Autodesk Inventor part; units mm, degrees
ref_plane "YZ Plane" through (0, 0, 0) normal (1, 0, 0) x (0, 1, 0)
ref_plane "XZ Plane" through (0, 0, 0) normal (0, 1, 0) x (-1, 0, 0)
ref_plane "XY Plane" through (0, 0, 0) normal (0, 0, 1) x (1, 0, 0)
sketch "Boceto1" plane through (0, 0, 0) normal (0, 0, 1) x (1, 0, 0)
  line L0 (0, 0) -> (127.5, 0)
  line L1 (127.5, 0) -> (127.5, 177)
  line L2 (127.5, 177) -> (0, 177)
  line L3 (0, 177) -> (0, 0)
  dimension "d32" = 127.5
  dimension "d33" = 177
extrude "Extrusión1" add sketch "Boceto1" along normal blind 6
ref_plane "Plano de trabajo6" through (0, 88.5, 0) normal (0, -1, 0) x (1, 0, 0)
ref_plane "Plano de trabajo7" through (63.75, 0, 0) normal (-1, 0, 0) x (0, 0, 1)
sketch "Boceto17" plane through (0, 0, 6) normal (0, 0, 1) x (1, 0, 0)
  line L0 (127.5, 0) -> (116, 0)
  line L1 (116, 0) -> (116, 11.5)
  line L2 (116, 11.5) -> (127.5, 11.5)
  line L3 (127.5, 11.5) -> (127.5, 0)
  line L4 (0, 0) -> (11.5, 0)
  line L5 (11.5, 0) -> (11.5, 11.5)
  line L6 (11.5, 11.5) -> (0, 11.5)
  line L7 (0, 11.5) -> (0, 0)
  line L8 (127.5, 177) -> (116, 177)
  line L9 (116, 177) -> (116, 165.5)
  line L10 (116, 165.5) -> (127.5, 165.5)
  line L11 (127.5, 165.5) -> (127.5, 177)
  line L12 (0, 177) -> (11.5, 177)
  line L13 (11.5, 177) -> (11.5, 165.5)
  line L14 (11.5, 165.5) -> (0, 165.5)
  line L15 (0, 165.5) -> (0, 177)
  dimension "d124" = 11.5
  dimension "d125" = 11.5
  dimension "d129" = 11.5
  dimension "d130" = 11.5
  dimension "d131" = 11.5
  dimension "d132" = 11.5
  dimension "d133" = 11.5
  dimension "d134" = 11.5
extrude "Extrusión12" cut sketch "Boceto17" against normal blind 4
sketch "Boceto18" plane through (0, 0, 2) normal (0, 0, 1) x (1, 0, 0)
  line L0 (0, 0) -> (11.5, 0)
  line L1 (11.5, 0) -> (11.5, 11.5)
  line L2 (11.5, 11.5) -> (0, 11.5)
  line L3 (0, 11.5) -> (0, 0)
  line L4 (127.5, 0) -> (116, 0)
  line L5 (116, 0) -> (116, 11.5)
  line L6 (116, 11.5) -> (127.5, 11.5)
  line L7 (127.5, 11.5) -> (127.5, 0)
  line L8 (127.5, 177) -> (116, 177)
  line L9 (116, 177) -> (116, 165.5)
  line L10 (116, 165.5) -> (127.5, 165.5)
  line L11 (127.5, 165.5) -> (127.5, 177)
  line L12 (0, 177) -> (11.5, 177)
  line L13 (11.5, 177) -> (11.5, 165.5)
  line L14 (11.5, 165.5) -> (0, 165.5)
  line L15 (0, 165.5) -> (0, 177)
  line L16 (116, 11.5) -> (127.5, 0)
  line L17 (127.5, 11.5) -> (116, 0)
  circle A0 centre (121.75, 5.75) radius 2
  dimension "d137" = 4
extrude "Extrusión13" cut sketch "Boceto18" against normal blind 3.2 contours A0 L17 L16 | L16 L17 A0 | A0 L16 L17 | L17 L16 A0
mirror "Simetría7" about plane through (63.75, 0, 0) normal (-1, 0, 0) of "Extrusión13"
mirror "Simetría8" about plane through (0, 88.5, 0) normal (0, -1, 0) of "Extrusión13", "Simetría7"
sketch "Boceto19" plane through (0, 0, 6) normal (0, 0, 1) x (1, 0, 0)
  line L0 (0, 0) -> (127.5, 0)
  line L1 (127.5, 0) -> (127.5, 85.5)
  line L2 (127.5, 85.5) -> (0, 85.5)
  line L3 (0, 85.5) -> (0, 0)
  line L4 (127.5, 0) -> (127.5, 177)
  line L5 (0, 85.5) -> (127.5, 85.5)
  line L6 (127.5, 85.5) -> (127.5, 91.5)
  line L7 (127.5, 91.5) -> (0, 91.5)
  line L8 (0, 91.5) -> (0, 85.5)
  line L9 (0, 91.5) -> (127.5, 91.5)
  line L10 (127.5, 91.5) -> (127.5, 177)
  line L11 (127.5, 177) -> (0, 177)
  line L12 (0, 177) -> (0, 91.5)
  dimension "d140" = 127.5
  dimension "d141" = 85.5
  dimension "d142" = 6
extrude "Extrusión14" cut sketch "Boceto19" against normal blind 4.2 contours L8 L7 L4 L2
properties part number "transillum_diffusor_partC_v1"
The listing builds one solid part. Answer for the finished solid, in the listing's coordinates (mm). A direction names the side the tool comes from. Give positions to 0.01 mm unless a question says otherwise; leave off trailing zeros. Write each loop counter-clockwise with the first axis right and the second up, starting at its lowest first coordinate (ties: lowest second). Pieces come first, ordered by that corner, then holes. Notation, with made-up numbers: (-21.75, -28) -> (3.25, -28) arc R17 ccw to (3.25, -22) -> close; hole circle Ø10 at (14.25, 0). An arc over 180 degrees is marked (long way). Use one line per item in the form item = value.
1) Section A-A on z = 4.8 is taken. Write down the section's boundary in (x, y), plus the area to 3 significant figures.
Result:
outline = (0, 11.5) -> (11.5, 11.5) -> (11.5, 0) -> (116, 0) -> (116, 11.5) -> (127.5, 11.5) -> (127.5, 85.5) -> (0, 85.5) -> close; (0, 91.5) -> (127.5, 91.5) -> (127.5, 165.5) -> (116, 165.5) -> (116, 177) -> (11.5, 177) -> (11.5, 165.5) -> (0, 165.5) -> close
area = 21,300 mm²
2) Each of these flat-tipped pins is pushed along its axis until it touches: P1, Ø2.5, axis at x = 121.75, y = 5.75, coming from the -Z side; P2, Ø2, axis at y = 172, z = 5, coming from the +X side; P3, Ø3, axis at x = 65, y = 111.5, coming from the -Z side; P4, Ø3.5, axis at x = 124, y = 8, coming from the +Z side. Where does it stop, or does it pass through?
Result:
P1 = through
P2 = 116
P3 = 0
P4 = 2
3) For a pull along Y with two mould halves and no side action, classify faces 1 (the flat face through (122, 165.5, 4)), 2 (the flat face through (119, 171, 2)), 3 (the flat face through (63, 89, 1.8)), 4 (the cylindrical face through (119.752, 5.838, 1.014)) as +Y half, -Y half, draft (parallel to the pull), parting line (faces both ways), or undercut.
Result:
face_1 = +Y half
face_2 = draft
face_3 = undercut
face_4 = undercut
4) Section C-C on x = 121.75 is taken. Write down the section's boundary in (y, z), plus the area to 3 significant figures.
Result:
outline = (0, 0) -> (3.75, 0) -> (3.75, 2) -> (0, 2) -> close; (7.75, 0) -> (169.25, 0) -> (169.25, 2) -> (165.5, 2) -> (165.5, 6) -> (91.5, 6) -> (91.5, 1.8) -> (85.5, 1.8) -> (85.5, 6) -> (11.5, 6) -> (11.5, 2) -> (7.75, 2) -> close; (173.25, 0) -> (177, 0) -> (177, 2) -> (173.25, 2) -> close
area = 929 mm²
5) Section B-B on y = 5.75 is taken. Write down the section's boundary in (x, z).
Result:
outline = (0, 0) -> (3.75, 0) -> (3.75, 2) -> (0, 2) -> close; (7.75, 0) -> (119.75, 0) -> (119.75, 2) -> (116, 2) -> (116, 6) -> (11.5, 6) -> (11.5, 2) -> (7.75, 2) -> close; (123.75, 0) -> (127.5, 0) -> (127.5, 2) -> (123.75, 2) -> close
6) A tool of negligible diameter and unlimited length cuts with its end or side. For faces 5 (the flat face through (6, 11.5, 4)), 6 (the flat face through (6, 165.5, 4)), 7 (the flat face through (122, 11.5, 4)), 8 (the flat face through (65, 85.5, 4)), from which of +Z, -Z, +X, -X, +Y, -Y can it reach the whole face along a straight path? Write none if from no direction.
Result:
face_5 = +Z, -X, -Y
face_6 = +Z, -X, +Y
face_7 = +Z, +X, -Y
face_8 = +Z, +X, -X
7) Straight lines are drawn through the part: probe 1 along X at (y, z) = (171.25, 0.95); probe 2 along Y at (x, z) = (121.75, 0.7); probe 3 along Y at (x, z) = (39.5, 2.95). For each, find the intervals that lie inside material, in ascending order.
Result:
probe_1 = 0 to 3.75, 7.75 to 119.75, 123.75 to 127.5
probe_2 = 0 to 3.75, 7.75 to 169.25, 173.25 to 177
probe_3 = 0 to 85.5, 91.5 to 177
8) Section D-D on x = 71 is taken. Write down the section's boundary in (y, z).
Result:
outline = (0, 0) -> (177, 0) -> (177, 6) -> (91.5, 6) -> (91.5, 1.8) -> (85.5, 1.8) -> (85.5, 6) -> (0, 6) -> close
